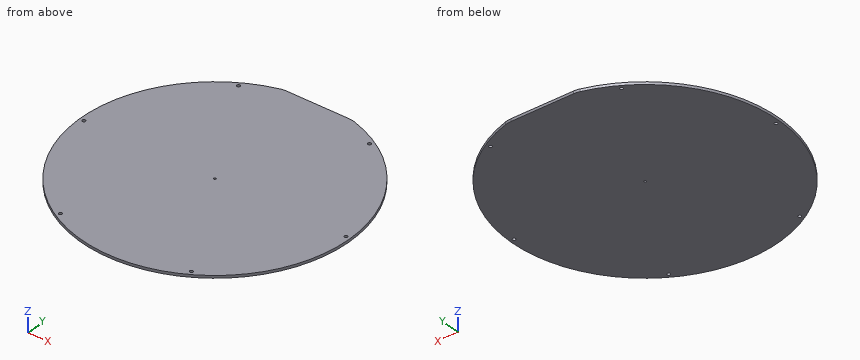
```python
from build123d import *

# Parameters (mm, degrees)
SKETCH1_R               = 155
SKETCH1_R_2             = 1.25
BOSS_EXTRUDE1_DEPTH     = 3
SKETCH2_R               = 1.85
CUT_EXTRUDE1_DEPTH      = 220.223630113
CIRPATTERN1_COUNT       = 6
CUT_EXTRUDE2_DEPTH      = 220.223630113
CUT_EXTRUDE2_DEPTH_BACK = 220.223630113
FILLET1_R               = 25


with BuildPart() as part:
    # Sketch1 → Boss-Extrude1 (new body)
    with BuildSketch(Plane.XY):
        Circle(SKETCH1_R)
        Circle(SKETCH1_R_2, mode=Mode.SUBTRACT)
    extrude(amount=BOSS_EXTRUDE1_DEPTH)

    # Sketch2 → Cut-Extrude1 (cut, through all)
    with BuildSketch(Plane.XY.offset(3)):
        with Locations((-150, 0)):
            Circle(SKETCH2_R)
    cut_extrude1 = extrude(amount=-CUT_EXTRUDE1_DEPTH, mode=Mode.SUBTRACT)

    # CirPattern1: Cut-Extrude1 ×6 about axis
    cirpattern1_axis = Axis((0, 0, 0), (0, 0, 1))
    for i in range(1, CIRPATTERN1_COUNT):
        add(cut_extrude1.rotate(cirpattern1_axis, i * 360 / CIRPATTERN1_COUNT), mode=Mode.SUBTRACT)

    # Sketch18 → Cut-Extrude2 (cut, two sides: drawn at the far end of the back side and taken through both)
    with BuildSketch(Plane.XY.offset(3).offset(-CUT_EXTRUDE2_DEPTH_BACK)):
        Polygon((-816.796213875, 150), (-60.219206673, 150), (46.353365048, 150), (802.93037225, 150), (802.93037225, 1663.154014405), (-816.796213875, 1663.154014405), align=None)
    extrude(amount=CUT_EXTRUDE2_DEPTH + CUT_EXTRUDE2_DEPTH_BACK, mode=Mode.SUBTRACT)

    # Fillet1
    fillet1_edges = [part.edges().sort_by_distance(p)[0] for p in [
        (-39.05124838, 150, 1.5),
        (39.05124838, 150, 1.5),
    ]]
    fillet(fillet1_edges, radius=FILLET1_R)


solid = part.part
```
Source: CAD feature listing. Evaluate the final solid. Frame: model axes, mm. Round coordinates to 2 decimals unless told otherwise and drop trailing zeros. Loops run counter-clockwise (first coordinate to the right, second up) from the corner with the lowest first, then second, coordinate; pieces in that order, holes last.
1. Section query B-B on y = 49. Output: boundary loops of the cut face in (x, z).
2. Section query C-C on x = 64. Output: boundary loops of the cut face in (y, z).
3. Section query A-A on z = 1.8. Output: boundary loops of the cut face in (x, y) (3 decimals), and give its area (3 significant figures).
4. Contact query for a flat-ended pin moving along its axis: pin 1 (1.5 mm diameter, centred on y = 35.5, z = 1.5, fed in from -X). Output: stop coordinate, or through.
5. Ray query, L1, parallel to X at y = 84.5, z = 1.95; L2, parallel to X at y = -125, z = 0.9; L3, parallel to Y at x = 132, z = 1.85. Return the intervals inside material, ascending.
Answers below:
1. outline: (-147.05, 0) - (147.05, 0) - (147.05, 3) - (-147.05, 3) - close
2. outline: (-141.17, 0) - (141.17, 0) - (141.17, 3) - (-141.17, 3) - close
3. outline: (-42.574, 149.038) arc R155 ccw (long way) to (42.574, 149.038) arc R25 ccw to (35.707, 150) - (-35.707, 150) arc R25 ccw to start; hole circle Ø3.7 at (-150, 0); hole circle Ø3.7 at (-75, -129.904); hole circle Ø3.7 at (-75, 129.904); hole circle Ø2.5 at (0, 0); hole circle Ø3.7 at (75, -129.904); hole circle Ø3.7 at (75, 129.904); hole circle Ø3.7 at (150, 0)
3. area: 75,100 mm2
4. pin 1: stops at x = -151.05
5. L1: x = -129.94 to 129.94
5. L2: x = -91.65 to 91.65
5. L3: y = -81.25 to 81.25
